Here's how the part is built. I have some questions about the finished solid (model axes, mm). A direction names the side the tool comes from. Coordinates: 2 decimals unless noted, no trailing zeros. Order: outer loops, then holes, each group sorted by start corner. A loop starts at its lowest first (then second) coordinate and runs counter-clockwise, first axis right, second up. Notation, with made-up numbers: M 62.25,5.25 L 93.25,5.25 A16 cw 93.25,18.25 Z; hole C 37.5,45 d4. An arc over 180 degrees is marked long. Answer as CSV lines item,"result". Start each with the question number.
Autodesk Inventor part; units mm, degrees
ref_plane "YZ Plane" through (0, 0, 0) normal (1, 0, 0) x (0, 1, 0)
ref_plane "XZ Plane" through (0, 0, 0) normal (0, 1, 0) x (-1, 0, 0)
ref_plane "XY Plane" through (0, 0, 0) normal (0, 0, 1) x (1, 0, 0)
sketch "Sketch1" plane through (0, 0, 0) normal (0, 1, 0) x (-1, 0, 0)
  line L0 (29, -17.5) -> (-29, -17.5)
  line L1 (-29, -17.5) -> (-29, 17.5)
  line L2 (-29, 17.5) -> (29, 17.5)
  line L3 (29, 17.5) -> (29, -17.5)
  line L4 (29, -17.5) -> (-29, 17.5) construction
  line L5 (-29, -17.5) -> (29, 17.5) construction
  point P0 (0, 0)
  dimension "d0" = 58
  dimension "d1" = 35
extrude "Extrusion1" add sketch "Sketch1" along normal blind 12.7
sketch "Sketch2" plane through (0, 0, 0) normal (0, -1, 0) x (1, 0, 0)
  line L0 (-29, -17.5) -> (29, -17.5)
  line L1 (29, -17.5) -> (29, 17.5)
  line L2 (29, 17.5) -> (-29, 17.5)
  line L3 (-29, 17.5) -> (-29, -17.5)
  line L4 (-24, 17.5) -> (-24, -17.5)
  line L5 (24, 17.5) -> (24, -17.5)
  point P0 (0, 0)
  dimension "d4" = 5
  dimension "d5" = 5
extrude "Extrusion2" add sketch "Sketch2" along normal blind 9.525 contours L3 L2 L4 L0 | L5 L2 L1 L0
sketch "Sketch3" plane through (0, 12.7, 0) normal (0, 1, 0) x (1, 0, 0)
  line L0 (29, 17.5) -> (-29, 17.5)
  line L1 (-29, 17.5) -> (-29, -17.5)
  point P0 (0, 0)
  point P1 (-19, 11)
  point P2 (19, 11)
  point P3 (-19, -11)
  point P4 (19, -11)
  dimension "d10" = 38
  dimension "d13" = 22
  dimension "d16" = 10
  dimension "d17" = 58
  dimension "d18" = 35
  dimension "d19" = 6.5
hole "Hole1" at (-19, 12.7, -11) at (19, 12.7, -11) at (-19, 12.7, 11) at (19, 12.7, 11) direction (0, -1, 0) diameter 5.25 end through all
equation "\"d5\" = d4"
properties part number "hd16_standoff"
1) Suppose I cut it at D-D on y = 3.5. Please give me the cut outline in (x, z) (3 decimals), plus the area to 3 significant figures.
2) Will these pins go through, and if not, where does the flat tip stop? pin 1 Ø6 at (x, z) = (-19, 11) entering from -Y; pin 2 Ø4 at (x, z) = (-19, -11) entering from +Y; pin 3 Ø6 at (x, z) = (19, -11) entering from +Y.
3) If we mould it in two halves opening along Z, with no side actions, what happens to faces 1 (the face through (-27, -9.525, 0)), 2 (the face through (0, 4, -17.5)), 3 (the face through (18.885, 6.261, 8.378)), 4 (the face through (0, 4, 17.5))? For each: released by +Z, released by -Z, zero draft, split by the parting line, or undercut.
4) Suppose I cut it at A-A on x = -19. Please give me the cut outline in (y, z) (3 decimals).
5) I need wall thicknesses on line 1 (Z direction, x = 19, y = 3.75) (3 decimals); line 2 (X direction, y = 9.75, z = -11) (3 decimals); line 3 (X direction, y = -2.5, z = -3). Which ranges of each line are inside material? Lowest first, please. Write a range as [from, to].
6) Suppose I cut it at B-B on y = -5.25. Please give me the cut outline in (x, z).
7) Suppose I cut it at C-C on z = 11. Please give me the cut outline in (x, y) (3 decimals), plus the area to 4 significant figures.
8) Which directions (+Z, -Z, +X, -X, +Y, -Y) give clear straight access to the entire face, cutting with the end or side of a thin tool? Please do faces 5 (the face through (0, 0, 0)), 6 (the face through (-20.774, 6.261, -12.935)).
Output:
1,outline,"M -29,-17.5 L 29,-17.5 L 29,17.5 L -29,17.5 Z; hole C -19,-11 d5.25; hole C -19,11 d5.25; hole C 19,-11 d5.25; hole C 19,11 d5.25"
1,area,"1,940 mm²"
2,pin 1,"y = 0"
2,pin 2,"through"
2,pin 3,"y = 12.7"
3,face 1,"zero draft"
3,face 2,"released by -Z"
3,face 3,"undercut"
3,face 4,"released by +Z"
4,outline,"M 0,-17.5 L 12.7,-17.5 L 12.7,-13.625 L 0,-13.625 Z; M 0,-8.375 L 12.7,-8.375 L 12.7,8.375 L 0,8.375 Z; M 0,13.625 L 12.7,13.625 L 12.7,17.5 L 0,17.5 Z"
5,line 1,"[-17.5, -13.625], [-8.375, 8.375], [13.625, 17.5]"
5,line 2,"[-29, -21.625], [-16.375, 16.375], [21.625, 29]"
5,line 3,"[-29, -24], [24, 29]"
6,outline,"M -29,-17.5 L -24,-17.5 L -24,17.5 L -29,17.5 Z; M 24,-17.5 L 29,-17.5 L 29,17.5 L 24,17.5 Z"
7,outline,"M -29,-9.525 L -24,-9.525 L -24,0 L -21.625,0 L -21.625,12.7 L -29,12.7 Z; M -16.375,0 L 16.375,0 L 16.375,12.7 L -16.375,12.7 Z; M 21.625,0 L 24,0 L 24,-9.525 L 29,-9.525 L 29,12.7 L 21.625,12.7 Z"
7,area,"698.5 mm²"
8,face 5,"+Z, -Z, -Y"
8,face 6,"+Y, -Y"
